from build123d import *

# Parameters (mm, degrees)
BOSS_EXTRUDE8_DEPTH  = 46.84
SKETCH10_R           = 5
BOSS_EXTRUDE9_DEPTH  = 5
SKETCH11_R           = 2.5
CUT_EXTRUDE4_DEPTH   = 94.68
BOSS_EXTRUDE10_DEPTH = 5


with BuildPart() as part:
    # Sketch9 → Boss-Extrude8 (new body, symmetric)
    with BuildSketch(Plane(origin=(0, 0, 0), x_dir=(0, 0, -1), z_dir=(1, 0, 0))):
        with BuildLine():
            Line((0, 0), (-0.173648178, 0.984807753))
            ThreePointArc((-0.173648178, 0.984807753), (-22.828245747, 74.423796966), (-62.906637971, 140))
            ThreePointArc((-62.906637971, 140), (-66.419974037, 140.395562491), (-66.815536529, 136.882226425))
            ThreePointArc((-66.815536529, 136.882226425), (-27.385689632, 72.367172247), (-5.097686943, 0.116566865))
            Line((-5.097686943, 0.116566865), (-5.077133059, 0))
            Line((-5.077133059, 0), (0, 0))
        make_face()
    extrude(amount=BOSS_EXTRUDE8_DEPTH, both=True)

    # Sketch10 → Boss-Extrude9 (add)
    with BuildSketch(Plane(origin=(46.84, 0, 0), x_dir=(0, 0, -1), z_dir=(1, 0, 0))):
        with Locations((-5.077133059, 0)):
            Circle(SKETCH10_R)
    boss_extrude9 = extrude(amount=-BOSS_EXTRUDE9_DEPTH)

    # Mirror1: Boss-Extrude9 across plane
    add(boss_extrude9.mirror(Plane(origin=(0, 0, 0), x_dir=(0, 0, 1), z_dir=(1, 0, 0))))

    # Sketch11 → Cut-Extrude4 (cut, through all)
    with BuildSketch(Plane(origin=(46.84, 0, 0), x_dir=(0, 0, -1), z_dir=(1, 0, 0))):
        with Locations((-5.077133059, 0)):
            Circle(SKETCH11_R)
    extrude(amount=-CUT_EXTRUDE4_DEPTH, mode=Mode.SUBTRACT)

    # Sketch13 → Boss-Extrude10 (add)
    with BuildSketch(Plane(origin=(46.84, 0, 0), x_dir=(0, 0, -1), z_dir=(1, 0, 0))):
        with BuildLine():
            Line((-10.077133059, 0), (-67.36108725, 0))
            Line((-67.36108725, 0), (-67.36108725, 138.441113213))
            ThreePointArc((-67.36108725, 138.441113213), (-67.220761295, 137.615317595), (-66.815536529, 136.882226425))
            ThreePointArc((-66.815536529, 136.882226425), (-28.39859142, 74.587920976), (-5.983948215, 4.917081072))
            ThreePointArc((-5.983948215, 4.917081072), (-8.919923438, 3.198900141), (-10.077133059, 0))
        make_face()
    extrude(amount=-BOSS_EXTRUDE10_DEPTH)


solid = part.part
Can you work these out from the model? Positions are in its coordinate system, mm. A direction names the side the tool comes from. Coordinates: 2 decimals unless noted, no trailing zeros. Loops run counter-clockwise (first coordinate to the right, second up) from the corner with the lowest first, then second, coordinate; pieces in that order, holes last. Notation, with made-up numbers: (-28.75, 35.25) - (23.25, 35.25) arc R22 cw to (23.25, 51.25) - close; hole circle Ø11 at (-8.5, 1). An arc over 180 degrees is marked (long way). Answer as a JSON object with one key per item and string values. Group by question number.
Item 1: If we section it at A-A (x = -31): List the corners of the cut face in (y, z) for me, plus the area to 3 significant figures.
Item 2: For pin 1 (8 mm diameter, centred on x = -5.5, z = 28, fed in from +Y); pin 2 (4 mm diameter, centred on x = 45, z = 36, fed in from -Y); pin 3 (4 mm diameter, centred on x = -29, z = 29, fed in from +Y), each with a flat end and sliding along its axis, tell me the tip position at first contact or that it passes through.
Item 3: On a 3-axis mill with a long thin cutter (end or side, diameter ignored), from which of +Z, -Z, +X, -X, +Y, -Y can I reach the whole of each face in a straight line? I mean faces 1 (the face through (-41.84, -2, 7)), 2 (the face through (0.656, 140.429, 66.377)), 3 (the face through (44, 0, 38)). Say none if no direction works.
Item 4: If we section it at B-B (y = 29): List the corners of the cut face in (x, z) for me, plus the area to 4 significant figures.
Item 5: If I drill on L1, parallel to X at y = 25.5, z = 31; L2, parallel to Z at x = 12, y = 77; L3, parallel to Z at x = -18.5, y = 116, over which ranges is the centre line in solid material (lowest first)? Write a range as from..to.
Item 6: If we mould it in two halves opening along Y, with no side actions, what happens to faces 4 (the face through (41.84, 52, 41)), 5 (the face through (-44.375, -3.739, 8.396)), 6 (the face through (44, -5, 5))? For each: released by +Y, released by -Y, zero draft, split by the parting line, or undercut.
Returned:
{
 "1": {"outline": "(0, 0) - (0.98, 0.17) arc R308.99 ccw to (140, 62.91) arc R2.5 ccw to (136.88, 66.82) arc R303.99 cw to (2.46, 5.52) arc R2.5 cw to (0, 2.58) - close", "area": "771 mm²"},
 "2": {"pin 1": "stops at y = 93.05", "pin 2": "stops at y = 0", "pin 3": "stops at y = 91.17"},
 "3": {"face 1": "+Z, -Y", "face 2": "-X", "face 3": "+Z, +X, -X, -Y"},
 "4": {"outline": "(-46.84, 6.47) - (46.84, 6.47) - (46.84, 67.36) - (41.84, 67.36) - (41.84, 11.66) - (-46.84, 11.66) - close", "area": "764.5 mm²"},
 "5": {"L1": "x = 41.84..46.84", "L2": "z = 24.01..29.52", "L3": "z = 45.58..51.57"},
 "6": {"face 4": "zero draft", "face 5": "undercut", "face 6": "released by -Y"}
}
